```python
from build123d import *

# Parameters (mm, degrees)
F0_R     = 1.97485
F1_DEPTH = 9.0932
F2_SIZE2 = 0.254
F2_SIZE  = 0.254
F3_SIZE2 = 0.254
F3_SIZE  = 0.254


with BuildPart() as f1:
    # F0 (on Right) → F1 (new body)
    with BuildSketch(Plane.YZ):
        Circle(F0_R)
    extrude(amount=-F1_DEPTH)

    # F2
    f2_edges = [f1.edges().sort_by_distance(p)[0] for p in [
        (0, -1.97485, 0),
    ]]
    chamfer(f2_edges, length=F2_SIZE, length2=F2_SIZE2)

    # F3
    f3_edges = [f1.edges().sort_by_distance(p)[0] for p in [
        (-9.0932, -1.97485, 0),
    ]]
    chamfer(f3_edges, length=F3_SIZE, length2=F3_SIZE2)


solid = f1.part
```
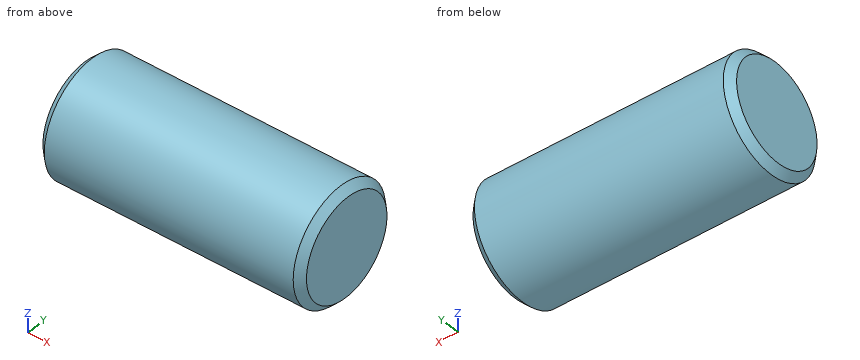
Input: part model. Units: mm. Frame: model coordinates. Coordinates: 2 decimals unless noted, no trailing zeros. Write each loop counter-clockwise with the first axis right and the second up, starting at its lowest first coordinate (ties: lowest second). Pieces come first, ordered by that corner, then holes. Notation, with made-up numbers: (8, 59) -> (12, 59) arc R32 cw to (12, 88) -> close; hole circle Ø7 at (-8.5, 22). An arc over 180 degrees is marked (long way). Answer as a JSON object with one key per item and string values.
1. Section A-A on x = -4.25. Return the cut outline in (y, z), then the cut area to 3 significant figures.
Result set:
{"outline": "circle Ø3.95 at (0, 0)", "area": "12.3 mm2"}
2. Material intervals for line 1 (Z direction, x = -1.5, y = -1.15); line 2 (Z direction, x = -7.5, y = 1); line 3 (Y direction, x = -3, z = 1.65), sorted ascending. Write a range as from..to.
Result set:
{"line 1": "z = -1.61..1.61", "line 2": "z = -1.7..1.7", "line 3": "y = -1.09..1.09"}
3. First-contact query: P1, Ø1, axis at x = -6, y = 1.5, coming from the -Z side. Flat tip, straight axial feed; report the tip coordinate or a pass-through.
Result set:
{"P1": "stops at z = -1.7"}
